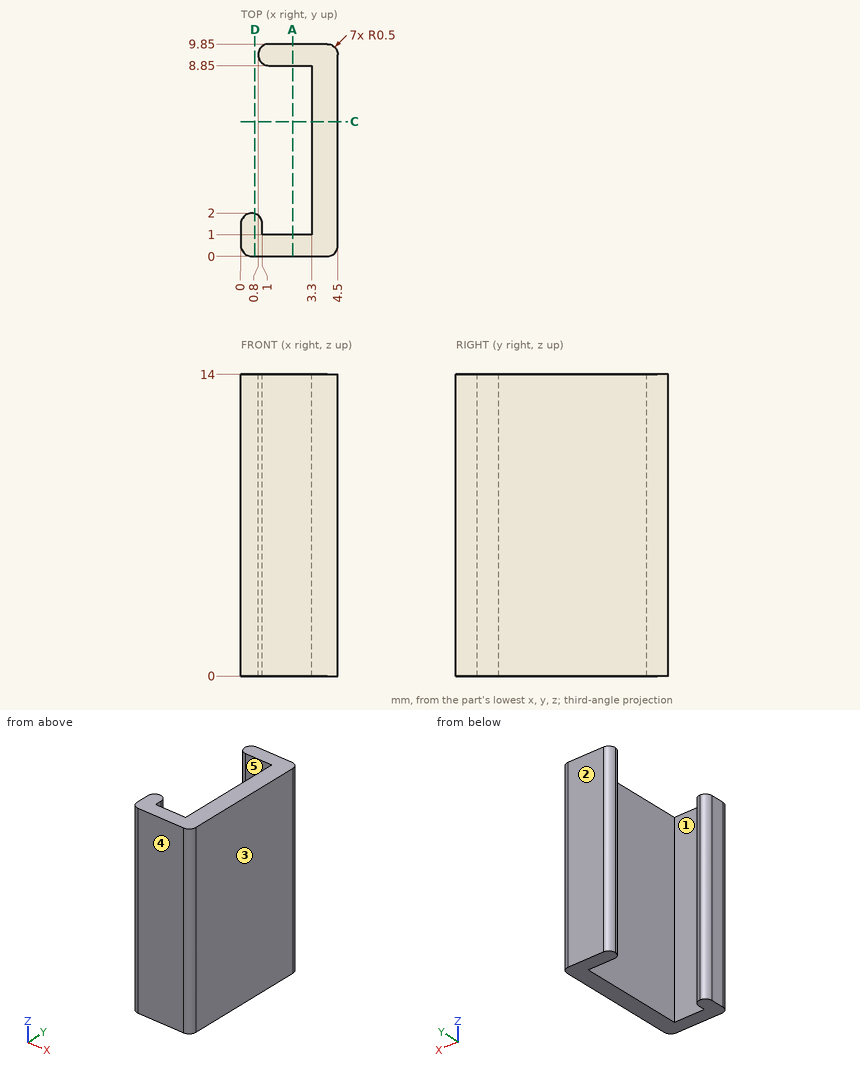
The drawing under review shows one solid part. Ordinate dimensions are in mm from its lowest x, y, z. A direction names the side the tool comes from. Coordinates: 2 decimals unless noted, no trailing zeros. Write each loop counter-clockwise with the first axis right and the second up, starting at its lowest first coordinate (ties: lowest second). Pieces come first, ordered by that corner, then holes. Notation, with made-up numbers: M -21,3 L 14,3 A27 cw 14,33 Z; hole C 39.5,-11 d10. An arc over 180 degrees is marked long. Answer as a JSON object with one key per item and string values.
Item 1: Add section A-A, the plane x = 2.4. Give the boundary of the cut face in (y, z).
Outcome:
{"outline": "M 0,0 L 1,0 L 1,14 L 0,14 Z; M 8.85,0 L 9.85,0 L 9.85,14 L 8.85,14 Z"}
Item 2: Add section D-D, the plane x = 0.65. Give the boundary of the cut face in (y, z).
Outcome:
{"outline": "M 0,0 L 1.98,0 L 1.98,14 L 0,14 Z"}
Item 3: Draft analysis for pull direction Y (two halves, no side actions). For the marked faces 1, 2 and 3, state which applies: pulls with the +Y half, pulls with the -Y half, needs draft (parallel to the pull), parting line crosses it, or undercut.
Outcome:
{"face 1": "undercut", "face 2": "pulls with the +Y half", "face 3": "needs draft"}
Item 4: Add section C-C, the plane y = 6.25. Give the boundary of the cut face in (x, z).
Outcome:
{"outline": "M 3.3,0 L 4.5,0 L 4.5,14 L 3.3,14 Z"}
Item 5: Machinability: for the marked faces 4 and 5, which of the approach directions +Z, -Z, +X, -X, +Y, -Y give a long, thin tool a straight path to every point of the face, cutting with its end or side? Answer none if there is none.
Outcome:
{"face 4": "+Z, -Z, +X, -X, -Y", "face 5": "+Z, -Z, -X"}
Item 6: Wall thickness on probe 1 along Y at (x, z) = (3.05, 12.25); probe 2 along X at (y, z) = (1.5, 8.75); probe 3 along Y at (x, z) = (0.45, 11.5): over which ranges is each line inside the solid? List them lowest first.
Outcome:
{"probe 1": "0 to 1, 8.85 to 9.85", "probe 2": "0 to 1, 3.3 to 4.5", "probe 3": "0 to 2"}
